Can you work these out from the model? Positions are in its coordinate system, mm. A direction names the side the tool comes from. Round coordinates to 2 decimals unless told otherwise and drop trailing zeros. Loops run counter-clockwise (first coordinate to the right, second up) from the corner with the lowest first, then second, coordinate; pieces in that order, holes last. Notation, with made-up numbers: M 8,-36 L 54,-36 A22 cw 54,-30 Z; hole C 15,-10 d6. An arc over 180 degrees is marked long. Use a Markdown table: item, result. Add a question column.
```python
from build123d import *


with BuildPart() as part:
    # Croquis1 → Revolución1 (revolve)
    with BuildSketch(Plane.XY):
        with BuildLine():
            Line((0, 0), (-5, 0))
            Line((-5, 0), (-3.850771176, 91.938305952))
            Line((-3.850771176, 91.938305952), (-3.334888704, 91.938305952))
            Line((-3.334888704, 91.938305952), (-3.334888704, 93.208903719))
            Line((-3.334888704, 93.208903719), (-3.834888704, 93.208903719))
            Line((-3.834888704, 93.208903719), (-3.819007472, 94.479402233))
            Line((-3.819007472, 94.479402233), (-3.303125, 94.479402233))
            Line((-3.303125, 94.479402233), (-3.303125, 95.75))
            Line((-3.303125, 95.75), (-3.803125, 95.75))
            Line((-3.803125, 95.75), (-3.75, 100))
            ThreePointArc((-3.75, 100), (-2.651650429, 102.651650429), (0, 103.75))
            Line((0, 103.75), (0, 100))
            Line((0, 100), (0, 0))
        make_face()
    revolve(axis=Axis((0, 100, 0), (0, -1, 0)))


solid = part.part
```
(1) Suppose I cut it at B-B on y = 13. List the corners of the cut face in (x, z) for me (1 decimal), and give its area (3 significant figures).
(2) If I drill on probe 1 along Z at (x, y) = (1.75, 97.5); probe 2 along Z at (x, y) = (3.25, 28); probe 3 along X at (y, z) = (89.5, -0.25), over which ranges is the centre line in solid material (lowest first)? Write a range as [from, to].
(3) I'm going to push flat-ended pins straight in: pin 1 (4 mm diameter, centred on y = 86, z = -1, fed in from +X); pin 2 (6 mm diameter, centred on x = 2.5, y = 81.5, fed in from -Z); pin 3 (3 mm diameter, centred on x = -0.5, z = -3, fed in from +Y). Where does each tip first touch, or does it pass through?
(4) Thinking about a two-plate mould opening in Y: for faces 1 (the face through (2, 94.479, -3)), 2 (the face through (0, 0, 0)), 3 (the face through (-1.74, 97.9, 3.35)), which applies, released by +Y, released by -Y, zero draft, split by the parting line, or undercut?
(5) On a 3-axis mill with a long thin cutter (end or side, diameter ignored), from which of +Z, -Z, +X, -X, +Y, -Y can I reach the whole of each face in a straight line? I mean faces 4 (the face through (-4.08, 46.61, 1.69)), 5 (the face through (3, 91.938, -2)). Say none if no direction works.
(6) Suppose I cut it at A-A on y = 64.5. List the corners of the cut face in (x, z) for me.
Results below:
| question | item | result |
|---|---|---|
| 1 | outline | C 0,0 d9.7 |
| 1 | area | 73.5 mm² |
| 2 | probe 1 | z = [-3.35, 3.35] |
| 2 | probe 2 | z = [-3.33, 3.33] |
| 2 | probe 3 | x = [-3.87, 3.87] |
| 3 | pin 1 | stops at x = 3.95 |
| 3 | pin 2 | stops at z = -4 |
| 3 | pin 3 | stops at y = 103.42 |
| 4 | face 1 | undercut |
| 4 | face 2 | released by -Y |
| 4 | face 3 | released by +Y |
| 5 | face 4 | +Y |
| 5 | face 5 | none |
| 6 | outline | C 0,0 d8.39 |
